Autodesk Inventor part; units mm, degrees
ref_plane "YZ Plane" through (0, 0, 0) normal (1, 0, 0) x (0, 1, 0)
ref_plane "XZ Plane" through (0, 0, 0) normal (0, 1, 0) x (-1, 0, 0)
ref_plane "XY Plane" through (0, 0, 0) normal (0, 0, 1) x (1, 0, 0)
sketch "Sketch_1" plane through (0, 0, 0) normal (0, 0, 1) x (1, 0, 0)
  line L0 (41, 0) -> (0, 0)
  line L1 (0, 8.92) -> (0, 3.27)
  arc A0 (0, 3.27) -> (0.77, 2.5) centre (0.77, 3.27) ccw
  line L2 (0.77, 2.5) -> (35, 2.5)
  line L3 (35, 2.5) -> (35, 10.2)
  arc A1 (39.1884, 6.3116) -> (35, 10.2) centre (35, 6) ccw
  arc A2 (39.1884, 6.3116) -> (41, 6) centre (40.225, 6.9162) ccw
  arc A3 (41, 6) -> (35, 12) centre (35, 6) ccw
  line L4 (35, 12) -> (33.5, 12)
  line L5 (33.5, 12) -> (29.5, 16)
  line L6 (29.5, 16) -> (23, 16)
  line L7 (23, 16) -> (23, 10.2)
  line L8 (23, 10.2) -> (14, 10.2)
  line L9 (14, 10.2) -> (14, 16)
  line L10 (14, 16) -> (9, 16)
  line L11 (9, 16) -> (9, 9.69)
  line L12 (9, 9.69) -> (7.2, 9.69)
  line L13 (7.2, 9.69) -> (6.3167, 10.2)
  line L14 (6.3167, 10.2) -> (0.9, 10.2)
  line L15 (0.9, 10.2) -> (0.9, 9.69)
  line L16 (0.9, 9.69) -> (0.77, 9.69)
  arc A4 (0.77, 9.69) -> (0, 8.92) centre (0.77, 8.92) ccw
revolve "Revolution1" add sketch "Sketch_1" angle 360 about axis through (41, 0, 0) along (-1, 0, 0)
sketch "Sketch_2" plane through (9, 0, 0) normal (1, 0, 0) x (0, 0, -1)
  line L0 (-24, 24) -> (-24, -24)
  line L1 (-24, -24) -> (24, -24)
  line L2 (24, -24) -> (24, 24)
  line L3 (24, 24) -> (-24, 24)
  arc A0 (-12, -5.6181) -> (-10.8654, -7.5833) centre (0, 0) ccw
  line L4 (-10.8654, -7.5833) -> (-1.1346, -13.2013)
  arc A1 (-1.1346, -13.2013) -> (1.1346, -13.2013) centre (0, 0) ccw
  line L5 (1.1346, -13.2013) -> (10.8654, -7.5833)
  arc A2 (10.8654, -7.5833) -> (12, -5.6181) centre (0, 0) ccw
  line L6 (12, -5.6181) -> (12, 5.6181)
  arc A3 (12, 5.6181) -> (10.8654, 7.5833) centre (0, 0) ccw
  line L7 (10.8654, 7.5833) -> (1.1346, 13.2013)
  arc A4 (1.1346, 13.2013) -> (-1.1346, 13.2013) centre (0, 0) ccw
  line L8 (-1.1346, 13.2013) -> (-10.8654, 7.5833)
  arc A5 (-10.8654, 7.5833) -> (-12, 5.6181) centre (0, 0) ccw
  line L9 (-12, 5.6181) -> (-12, -5.6181)
extrude "Extrusion1" cut sketch "Sketch_2" along normal blind 41
sketch "Skizze_1" plane through (0, 0, 12) normal (0, 0, 1) x (1, 0, 0)
  line L0 (9.6667, 1.8333) -> (9.6667, -1.8333)
  line L1 (9.6667, -1.8333) -> (13.3333, -1.8333)
  line L2 (13.3333, -1.8333) -> (13.3333, 1.8333)
  line L3 (13.3333, 1.8333) -> (9.6667, 1.8333)
  arc A0 (9.8713, 0.3539) -> (10.3904, -1.2436) centre (11.5, 0) ccw
  line L4 (10.3904, -1.2436) -> (10.4659, -1.1398)
  arc A1 (10.7355, -1.3357) -> (10.4659, -1.1398) centre (10.9122, -0.809) ccw
  line L5 (10.7355, -1.3357) -> (10.6601, -1.4396)
  arc A2 (10.6601, -1.4396) -> (12.3399, -1.4396) centre (11.5, 0) ccw
  line L6 (12.3399, -1.4396) -> (12.2645, -1.3357)
  arc A3 (12.5341, -1.1398) -> (12.2645, -1.3357) centre (12.0878, -0.809) ccw
  line L7 (12.5341, -1.1398) -> (12.6096, -1.2436)
  arc A4 (12.6096, -1.2436) -> (13.1287, 0.3539) centre (11.5, 0) ccw
  line L8 (13.1287, 0.3539) -> (13.0066, 0.3143)
  arc A5 (12.9036, 0.6313) -> (13.0066, 0.3143) centre (12.4511, 0.309) ccw
  line L9 (12.9036, 0.6313) -> (13.0256, 0.671)
  arc A6 (13.0256, 0.671) -> (11.6667, 1.6583) centre (11.5, 0) ccw
  line L10 (11.6667, 1.6583) -> (11.6667, 1.53)
  arc A7 (11.3333, 1.53) -> (11.6667, 1.53) centre (11.5, 1) ccw
  line L11 (11.3333, 1.53) -> (11.3333, 1.6583)
  arc A8 (11.3333, 1.6583) -> (9.9744, 0.671) centre (11.5, 0) ccw
  line L12 (9.9744, 0.671) -> (10.0964, 0.6313)
  arc A9 (9.9934, 0.3143) -> (10.0964, 0.6313) centre (10.5489, 0.309) ccw
  line L13 (9.9934, 0.3143) -> (9.8713, 0.3539)
extrude "Extrusion2" cut sketch "Skizze_1" against normal blind 0.048
properties part number "SKINTOP ST PG 13,5      Art. Nr. 53015030(F=5) Kunststoff"
Geometry: final body of the model. Coordinates: model frame, mm. A direction names the side the tool comes from. Round coordinates to 2 decimals unless told otherwise and drop trailing zeros. Loops run counter-clockwise (first coordinate to the right, second up) from the corner with the lowest first, then second, coordinate; pieces in that order, holes last.
Item 1: Mould query, pull axis X, two halves, no side actions, for faces 3 (the flat face through (11.5, 0.8, 11.952)), 4 (the flat face through (0.9, 9, 4)), 5 (the flat face through (11.465, 10.432, 5.932)). Classes: released by +X, released by -X, zero draft, split by the parting line, or undercut.
Checked values:
face 3: undercut
face 4: released by -X
face 5: zero draft
Item 2: Contact query for flat-ended pins moving along their axis: P1, Ø2, axis at x = 4.5, y = 7.5, coming from the +Z side; P2, Ø6, axis at x = 14.5, y = -10.5, coming from the -Z side; P3, Ø2, axis at x = 7.5, y = 6.5, coming from the +Z side. Output: stop coordinate, or through.
Checked values:
P1: stops at z = 7.86
P2: stops at z = -10.89
P3: stops at z = 8.06
Item 3: Section B-B, the plane x = 18. Output: boundary loops of the cut face in (y, z).
Checked values:
outline: circle Ø20.4 at (0, 0); hole circle Ø5 at (0, 0)
Item 4: Reachability of faces 1 (the cylindrical face through (3.57, 4.707, 9.049)), 2 (the flat face through (28, 0, 12)) from +Z, -Z, +X, -X, +Y, -Y: full face, straight path, thin tool, end or side. Return the list, or none.
Checked values:
face 1: -X
face 2: +Z, +X, -X, +Y, -Y
Item 5: Line query: L1, parallel to Y at x = 19, z = 0; L2, parallel to Y at x = 21, z = 1.5; L3, parallel to Z at x = 17.5, y = 1.75. Output: solid intervals per line, ascending.
Checked values:
L1: y = -10.2 to -2.5, 2.5 to 10.2
L2: y = -10.09 to -2, 2 to 10.09
L3: z = -10.05 to -1.79, 1.79 to 10.05
Item 6: Section A-A, the plane x = 25. Output: boundary loops of the cut face in (y, z), plus the area to 3 significant figures.
Checked values:
outline: (-13.2, -1.13) - (-7.58, -10.87) arc R13.25 ccw to (-5.62, -12) - (5.62, -12) arc R13.25 ccw to (7.58, -10.87) - (13.2, -1.13) arc R13.25 ccw to (13.2, 1.13) - (7.58, 10.87) arc R13.25 ccw to (5.62, 12) - (-5.62, 12) arc R13.25 ccw to (-7.58, 10.87) - (-13.2, 1.13) arc R13.25 ccw to start; hole circle Ø5 at (0, 0)
area: 475 mm2
